For this review, take the finished solid that the model builds, in its own axes (mm). A direction names the side the tool comes from. Round coordinates to 2 decimals unless told otherwise and drop trailing zeros. Loops run counter-clockwise (first coordinate to the right, second up) from the corner with the lowest first, then second, coordinate; pieces in that order, holes last.
1) Mouldability with a two-part tool opening along Y and no side actions: class faces 4 (the flat face through (-0.1, 9.5, 7.543)), 5 (the flat face through (9.5, 7, 7)), 6 (the flat face through (0, -10, 0)) as pulls with the +Y half, pulls with the -Y half, needs draft (parallel to the pull), parting line crosses it, or undercut.
2) Take a section at B-B (x = 6.5). State the section outline as (y, z) points.
3) Take a section at A-A (z = -6.75). State the section outline as (x, y) points.
4) Take a section at C-C (y = -5). State the section outline as (x, z) points, then the cut area to 3 significant figures.
5) Take a section at D-D (z = 6.25). State the section outline as (x, y) points, then the cut area to 3 significant figures.
6) Wall thickness on L1, parallel to Z at x = 9.25, y = 1.5; L2, parallel to X at y = -1, z = 0.5; L3, parallel to Y at x = 9.25, z = -5: over which ranges is each line inside the solid? List them lowest first.
7) Tool access review of faces 1 (the flat face through (-0.1, 9.5, -7.586)), 2 (the flat face through (9.507, 4.168, 2.754)), 3 (the flat face through (7, 7, 9.5)): name each direction out of +Z, -Z, +X, -X, +Y, -Y from which nothing blocks a thin tool from reaching the whole face with its end or side.
8) Insertion check: pin 1 (7 mm diameter, centred on x = 3, y = 2, fed in from +Z). The pin has a flat end and moves straight along its axis. Give the tip position at first contact, or say it passes through.
Autodesk Inventor part; units mm, degrees
ref_plane "YZ Plane" through (0, 0, 0) normal (1, 0, 0) x (0, 1, 0)
ref_plane "XZ Plane" through (0, 0, 0) normal (0, 1, 0) x (-1, 0, 0)
ref_plane "XY Plane" through (0, 0, 0) normal (0, 0, 1) x (1, 0, 0)
sketch "Esboço1" plane through (0, 0, 0) normal (0, 0, 1) x (1, 0, 0)
  line L0 (-10, -10) -> (10, -10)
  line L1 (10, -10) -> (10, 10)
  line L2 (10, 10) -> (-10, 10)
  line L3 (-10, 10) -> (-10, -10)
  line L4 (-10, -10) -> (10, 10) construction
  line L5 (10, -10) -> (-10, 10) construction
  point P0 (0, 0)
  dimension "d0" = 20
  dimension "d1" = 20
extrude "Extrusão1" add sketch "Esboço1" along normal mid plane 20
sketch "Esboço4" plane through (0, 0, 10) normal (0, 0, 1) x (1, 0, 0)
  line L0 (-7, -7) -> (7, -7) construction
  line L1 (7, -7) -> (7, 7) construction
  line L2 (7, 7) -> (-7, 7) construction
  line L3 (-7, 7) -> (-7, -7) construction
  line L4 (0, 1.4142) -> (-1.4142, 0)
  line L5 (-1.4142, 0) -> (0, -1.4142)
  line L6 (0, -1.4142) -> (1.4142, 0)
  line L7 (1.4142, 0) -> (0, 1.4142)
  line L8 (0, 1.4142) -> (0, -1.4142) construction
  line L9 (-1.4142, 0) -> (1.4142, 0) construction
  line L10 (0, -1.4142) -> (1.4142, 0)
  line L11 (1.4142, 0) -> (7.0002, -5.586)
  line L12 (5.586, -7.0002) -> (0, -1.4142)
  line L13 (0, -1.4142) -> (-1.4142, 0)
  line L14 (-1.4142, 0) -> (-7.0001, -5.5859)
  line L15 (-5.5859, -7.0001) -> (0, -1.4142)
  line L16 (-1.4142, 0) -> (0, 1.4142)
  line L17 (0, 1.4142) -> (-5.5858, 7)
  line L18 (-7, 5.5858) -> (-1.4142, 0)
  line L19 (1.4142, 0) -> (0, 1.4142)
  line L20 (0, 1.4142) -> (5.5858, 7)
  line L21 (7, 5.5858) -> (1.4142, 0)
  line L22 (-8.4142, 7) -> (-7, 5.5858)
  line L23 (7, 5.5858) -> (8.4142, 7)
  line L24 (8.4142, -7) -> (7, -5.5858)
  line L25 (-7, -5.5858) -> (-8.4142, -7)
  line L26 (-5.5858, -7) -> (-8.4142, -7)
  line L27 (5.5858, -7) -> (7, -7)
  line L28 (7, -7) -> (8.4142, -7)
  line L29 (-5.5858, 7) -> (-8.4142, 7)
  line L30 (5.5858, 7) -> (7, 7)
  line L31 (7, 7) -> (8.4142, 7)
  point P0 (0, 0)
  point P1 (0, 0)
  point P2 (-7, 7)
  point P3 (-7, -7)
  point P4 (6.2929, 7)
  point P5 (7.7071, -7)
  dimension "d62" = 2
  dimension "d63" = 2
  dimension "d64" = 14
  dimension "d65" = 14
  dimension "d68" = 2
  dimension "d69" = 2
  dimension "d70" = 2
  dimension "d71" = 2
extrude "Extrusão4" cut sketch "Esboço4" against normal blind 1
sketch "Esboço7" plane through (10, -10, 10) normal (1, 0, 0) x (0, 0, -1)
  line L0 (17, 3) -> (3, 3) construction
  line L1 (3, 3) -> (3, 17) construction
  line L2 (3, 17) -> (17, 17) construction
  line L3 (17, 17) -> (17, 3) construction
  line L4 (8.5858, 10) -> (10, 11.4142) construction
  line L5 (10, 11.4142) -> (11.4142, 10) construction
  line L6 (11.4142, 10) -> (11, 9.5858) construction
  line L7 (9, 9.5858) -> (8.5858, 10) construction
  line L8 (8.5858, 10) -> (11.4142, 10) construction
  line L9 (10, 11.4142) -> (10, 8.5858) construction
  line L10 (10, 11.4142) -> (4.4142, 17)
  line L11 (3, 15.5858) -> (8.5858, 10)
  line L12 (10, 11.4142) -> (15.5858, 17)
  line L13 (17, 15.5858) -> (11.4142, 10)
  line L14 (18.4142, 17) -> (17, 15.5858) construction
  line L15 (15.5858, 17) -> (18.4142, 17) construction
  line L16 (3, 15.5858) -> (1.5858, 17) construction
  line L17 (1.5858, 17) -> (4.4142, 17) construction
  line L18 (4.4142, 17) -> (1.5858, 17)
  line L19 (3, 15.5858) -> (1.5858, 17)
  line L20 (15.5858, 17) -> (18.4142, 17)
  line L21 (17, 15.5858) -> (18.4142, 17)
  line L22 (8.5858, 10) -> (9, 9.5858)
  line L23 (11.4142, 10) -> (11, 9.5858)
  line L24 (9, 3) -> (11, 3)
  line L25 (11, 3) -> (11, 9.5858)
  line L26 (9, 9.5858) -> (9, 3)
  line L27 (8.5858, 10) -> (10, 8.5858) construction
  line L28 (10, 8.5858) -> (11.4142, 10) construction
  point P0 (10, 10)
  point P1 (4.4142, 17)
  point P2 (8.7929, 9.7929)
extrude "Extrusão7" cut sketch "Esboço7" against normal blind 1
sketch "Esboço8" plane through (-10, 10, 10) normal (0, 1, 0) x (1, 0, 0)
  line L0 (17, 17.5858) -> (3, 17.5858) construction
  line L1 (10, 11.4142) -> (8.5858, 10) construction
  line L2 (8.5858, 10) -> (10, 8.5858) construction
  line L3 (10, 8.5858) -> (11.4142, 10) construction
  line L4 (11.4142, 10) -> (10, 11.4142) construction
  line L5 (10, 11.4142) -> (10, 8.5858) construction
  line L6 (8.5858, 10) -> (11.4142, 10) construction
  line L7 (11.4142, 10) -> (17, 15.5858)
  line L8 (14.1716, 15.5858) -> (10, 11.4142)
  line L9 (8.5858, 10) -> (3, 4.4142)
  line L10 (5.8712, 4.457) -> (10, 8.5858)
  line L11 (10, 11.4142) -> (8.5858, 10)
  line L12 (11.4142, 10) -> (10, 8.5858)
  line L13 (3, 4.4142) -> (3, 2.457)
  line L14 (17, 2.457) -> (17, 4.457)
  line L15 (17, 4.457) -> (5.8712, 4.457)
  line L16 (17, 17.5858) -> (17, 15.5858)
  line L17 (14.1716, 15.5858) -> (3, 15.5858)
  line L18 (3, 15.5858) -> (3, 17.5858)
  line L19 (3, 17.5858) -> (17, 17.5858)
  line L20 (3, 2.457) -> (17, 2.457)
  point P0 (10, 10)
extrude "Extrusão8" cut sketch "Esboço8" against normal blind 1
properties part number "Cubo-0001-002" material "Borracha"
Response:
1. face 4: needs draft
1. face 5: undercut
1. face 6: pulls with the -Y half
2. outline: (-10, -10) - (10, -10) - (10, -7.59) - (9, -7.59) - (9, -5.09) - (10, -5.09) - (10, 5.54) - (9, 5.54) - (9, 7.54) - (10, 7.54) - (10, 10) - (7, 10) - (7, 9) - (5.09, 9) - (5.09, 10) - (-5.09, 10) - (-5.09, 9) - (-7, 9) - (-7, 10) - (-10, 10) - close
3. outline: (-10, -10) - (10, -10) - (10, 5.34) - (9, 5.34) - (9, 7) - (10, 7) - (10, 10) - (7, 10) - (7, 9) - (-7, 9) - (-7, 10) - (-10, 10) - close
4. outline: (-10, -10) - (10, -10) - (10, -1) - (9, -1) - (9, 1) - (10, 1) - (10, 10) - (6.41, 10) - (6.41, 9) - (3.59, 9) - (3.59, 10) - (-3.59, 10) - (-3.59, 9) - (-6.41, 9) - (-6.41, 10) - (-10, 10) - close
4. area: 392 mm2
5. outline: (-10, -10) - (10, -10) - (10, 4.84) - (9, 4.84) - (9, 7) - (10, 7) - (10, 10) - (7, 10) - (7, 9) - (-7, 9) - (-7, 10) - (-10, 10) - close
5. area: 384 mm2
6. L1: z = -10 to -2.91, -0.09 to 0.09, 2.91 to 10
6. L2: x = -10 to 9
6. L3: y = -10 to 3.59, 6.41 to 10
7. face 1: +Y
7. face 2: +X
7. face 3: +Z
8. pin 1: stops at z = 10
